```python
from build123d import *

# Parameters (mm, degrees)
IZIM1_R                     = 25.75
Y_KSEKLIK_EKSTR_ZYON2_DEPTH = 22.56
IZIM2_R                     = 21.75
KES_EKSTR_ZYON1_DEPTH       = 22.56
IZIM3_R                     = 27.47
Y_KSEKLIK_EKSTR_ZYON3_DEPTH = 8
PAH1_SIZE                   = 4
Y_KSEKLIK_EKSTR_ZYON4_START = 8
IZIM5_R                     = 27.47
Y_KSEKLIK_EKSTR_ZYON4_DEPTH = 8
PAH2_SIZE                   = 4
IZIM6_R                     = 21.75
KES_EKSTR_ZYON4_DEPTH       = 8
KES_EKSTR_ZYON5_START       = -8
IZIM7_R                     = 21.75
KES_EKSTR_ZYON5_DEPTH       = 8
KES_EKSTR_ZYON6_START       = -64
KES_EKSTR_ZYON6_DEPTH       = 64


with BuildPart() as part:
    # Çizim1 → Yükseklik-Ekstrüzyon2 (new body)
    with BuildSketch(Plane.XY):
        Circle(IZIM1_R)
    extrude(amount=Y_KSEKLIK_EKSTR_ZYON2_DEPTH)

    # Çizim2 → Kes-Ekstrüzyon1 (cut)
    with BuildSketch(Plane.XY.offset(22.56)):
        Circle(IZIM2_R)
    extrude(amount=-KES_EKSTR_ZYON1_DEPTH, mode=Mode.SUBTRACT)

    # Çizim3 → Yükseklik-Ekstrüzyon3 (add)
    with BuildSketch(Plane.XY.offset(22.56)):
        Circle(IZIM3_R)
    extrude(amount=Y_KSEKLIK_EKSTR_ZYON3_DEPTH)

    # Pah1
    # the kernel refuses this chamfer: 4 mm, written as the material it takes off along each edge
    with BuildSketch(Plane(origin=(0, 0, 22.56), x_dir=(1, 0, 0), z_dir=(0, -1, 0))) as pah1_piece_1_section:
        Polygon((27.47, PAH1_SIZE), (27.47 - PAH1_SIZE, 0), (27.47, 0), align=None)
    pah1_piece_1 = revolve(axis=Axis((0, 0, 22.56), (0, 0, 1)), mode=Mode.PRIVATE)
    pah1_piece_1 = pah1_piece_1 - Plane(origin=(0, 0, 25.685965648), x_dir=(1, 0, 0), z_dir=(0, 0, -1)) * Cylinder(25.75, 110, mode=Mode.PRIVATE)
    add(pah1_piece_1, mode=Mode.SUBTRACT)

    # Çizim5 → Yükseklik-Ekstrüzyon4 (add)
    with BuildSketch(Plane(origin=(0, 0, 0), x_dir=(-1, 0, 0), z_dir=(0, 0, -1)).offset(Y_KSEKLIK_EKSTR_ZYON4_START)):
        with Locations(Location((0, 0, 0), (0, 0, 180))):
            Circle(IZIM5_R)
    extrude(amount=-Y_KSEKLIK_EKSTR_ZYON4_DEPTH)

    # Pah2
    # the kernel refuses this chamfer: 4 mm, written as the material it takes off along each edge
    with BuildSketch(Plane(origin=(0, 0, 0), x_dir=(1, 0, 0), z_dir=(0, 1, 0))) as pah2_piece_1_section:
        Polygon((27.47, PAH2_SIZE), (27.47 - PAH2_SIZE, 0), (27.47, 0), align=None)
    pah2_piece_1 = revolve(axis=Axis((0, 0, 0), (0, 0, -1)), mode=Mode.PRIVATE)
    pah2_piece_1 = pah2_piece_1 - Plane(origin=(0, 0, -3.125965648), x_dir=(1, 0, 0), z_dir=(0, 0, -1)) * Cylinder(25.75, 110, mode=Mode.PRIVATE)
    add(pah2_piece_1, mode=Mode.SUBTRACT)

    # Çizim6 → Kes-Ekstrüzyon4 (cut)
    with BuildSketch(Plane.XY.offset(30.56)):
        Circle(IZIM6_R)
    extrude(amount=-KES_EKSTR_ZYON4_DEPTH, mode=Mode.SUBTRACT)

    # Çizim7 → Kes-Ekstrüzyon5 (cut)
    with BuildSketch(Plane(origin=(0, 0, -8), x_dir=(-1, 0, 0), z_dir=(0, 0, -1)).offset(KES_EKSTR_ZYON5_START)):
        with Locations(Location((0, 0, 0), (0, 0, 180))):
            Circle(IZIM7_R)
    extrude(amount=KES_EKSTR_ZYON5_DEPTH, mode=Mode.SUBTRACT)

    # Çizim8 → Kes-Ekstrüzyon6 (cut)
    with BuildSketch(Plane(origin=(0, 0, -8), x_dir=(-1, 0, 0), z_dir=(0, 0, -1)).offset(KES_EKSTR_ZYON6_START)):
        with BuildLine():
            Line((21.728135562, 0.975), (27.45269158, 0.975))
            ThreePointArc((27.45269158, 0.975), (27.47, 0), (27.45269158, -0.975))
            Line((27.45269158, -0.975), (21.728135562, -0.975))
            ThreePointArc((21.728135562, -0.975), (21.75, 0), (21.728135562, 0.975))
        make_face()
    extrude(amount=KES_EKSTR_ZYON6_DEPTH, mode=Mode.SUBTRACT)


solid = part.part
```
Input: part model. Units: mm. Frame: model coordinates. A direction names the side the tool comes from. Give positions to 0.01 mm unless a question says otherwise; leave off trailing zeros. Order: outer loops, then holes, each group sorted by start corner. A loop starts at its lowest first (then second) coordinate and runs counter-clockwise, first axis right, second up.
1. Cut plane A-A (x = 0). Return loops of the section in (y, z).
Computed:
outline: (-27.47, -8) - (-21.75, -8) - (-21.75, 30.56) - (-27.47, 30.56) - (-27.47, 26.56) - (-25.75, 24.84) - (-25.75, -2.28) - (-27.47, -4) - close; (21.75, -8) - (27.47, -8) - (27.47, -4) - (25.75, -2.28) - (25.75, 24.84) - (27.47, 26.56) - (27.47, 30.56) - (21.75, 30.56) - close
2. Line query: probe 1 along Y at (x, z) = (0, -4); probe 2 along Y at (x, z) = (-16, 12.5); probe 3 along X at (y, z) = (-9, -1.5). Output: solid intervals per line, ascending.
Computed:
probe 1: y = -27.47 to -21.75, 21.75 to 27.47
probe 2: y = -20.18 to -14.73, 14.73 to 20.18
probe 3: x = -24.13 to -19.8, 19.8 to 24.13
3. Cut plane B-B (z = 11). Return loops of the section in (x, y) (3 decimals).
Computed:
outline: (-25.732, -0.975) arc R25.75 ccw (long way) to (-25.732, 0.975) - (-21.728, 0.975) arc R21.75 cw (long way) to (-21.728, -0.975) - close
4. Set-up query: faces 1 (the face through (0, -22, 30.56)), 2 (the face through (-24, 0.975, 12)). Return all of +Z, -Z, +X, -X, +Y, -Y with unobstructed straight access to the full face (end or side cutting, diameter ignored); none if empty.
Computed:
face 1: +Z, +X, -X, +Y, -Y
face 2: +Z, -Z, -X
5. Pin query (flat end, axial travel): pin 1 Ø8 at (x, z) = (21.5, 9) entering from +Y; pin 2 Ø6 at (x, z) = (19, 13) entering from -Y; pin 3 Ø6 at (x, z) = (-21, 10) entering from -Y. Return the tip coordinate at first contact, or that it passes through.
Computed:
pin 1: stops at y = 18.89
pin 2: stops at y = -20.18
pin 3: stops at y = -18.41
